```python
from build123d import *

# Parameters (mm, degrees)
BOSS_EXTRUDE1_DEPTH = 185
MIRROR3_START       = -185
MIRROR3_DEPTH       = 370


# Read off the part's stored shape, not the designer's step: Mirror3
with BuildPart() as part:
    # Sketch3 → Boss-Extrude1 (new, symmetric)
    with BuildSketch(Plane.XY):
        with BuildLine():
            Line((0, 8), (0, 3.5))
            ThreePointArc((0, 3.5), (-2.474873734, 2.474873734), (-3.5, 0))
            Line((-3.5, 0), (-8, 0))
            Line((-8, 0), (-8, 4.600266817))
            ThreePointArc((-8, 4.600266817), (-8.096672994, 5.086274776), (-8.371974388, 5.498292429))
            Line((-8.371974388, 5.498292429), (-13.873681959, 11))
            Line((-13.873681959, 11), (-17.7902, 11))
            Line((-17.7902, 11), (-17.7902, 6.2098))
            Line((-17.7902, 6.2098), (-17.0282, 6.2098))
            Line((-17.0282, 6.2098), (-17.0282, 4.508))
            ThreePointArc((-17.0282, 4.508), (-17.176989755, 4.148789755), (-17.5362, 4))
            Line((-17.5362, 4), (-18.8951, 4))
            ThreePointArc((-18.8951, 4), (-19.676382283, 4.323617717), (-20, 5.1049))
            Line((-20, 5.1049), (-20, 16.68))
            ThreePointArc((-20, 16.68), (-19.027594514, 19.027594514), (-16.68, 20))
            Line((-16.68, 20), (-5.1049, 20))
            ThreePointArc((-5.1049, 20), (-4.323617717, 19.676382283), (-4, 18.8951))
            Line((-4, 18.8951), (-4, 17.5362))
            ThreePointArc((-4, 17.5362), (-4.148789755, 17.176989755), (-4.508, 17.0282))
            Line((-4.508, 17.0282), (-6.2098, 17.0282))
            Line((-6.2098, 17.0282), (-6.2098, 17.7902))
            Line((-6.2098, 17.7902), (-11, 17.7902))
            Line((-11, 17.7902), (-11, 13.873681959))
            Line((-11, 13.873681959), (-5.498292429, 8.371974388))
            ThreePointArc((-5.498292429, 8.371974388), (-5.086274776, 8.096672994), (-4.600266817, 8))
            Line((-4.600266817, 8), (0, 8))
        make_face()
        with BuildLine():
            Line((-12.065, 18.73), (-12.065, 12.065))
            Line((-12.065, 12.065), (-18.73, 12.065))
            Line((-18.73, 12.065), (-18.73, 16.19))
            ThreePointArc((-18.73, 16.19), (-17.986051224, 17.986051224), (-16.19, 18.73))
            Line((-16.19, 18.73), (-12.065, 18.73))
        make_face(mode=Mode.SUBTRACT)
    extrude(amount=BOSS_EXTRUDE1_DEPTH, both=True)

    # Mirror1: part across plane


with BuildPart() as part_1:
    add(part.part)
    add(part.part.mirror(Plane(origin=(0, 0, 185), x_dir=(0, 0, 1), z_dir=(1, 0, 0))))

    # Mirror3 outline → Mirror3 (add)
    with BuildSketch(Plane.XY.offset(MIRROR3_START)):
        with BuildLine():
            Line((-8, 0), (-8, -4.600266817))
            ThreePointArc((-8, -4.600266817), (-8.096672994, -5.086274776), (-8.371974388, -5.498292429))
            Line((-8.371974388, -5.498292429), (-13.873681959, -11))
            Line((-13.873681959, -11), (-17.7902, -11))
            Line((-17.7902, -11), (-17.7902, -6.2098))
            Line((-17.7902, -6.2098), (-17.0282, -6.2098))
            Line((-17.0282, -6.2098), (-17.0282, -4.508))
            ThreePointArc((-17.0282, -4.508), (-17.176989755, -4.148789755), (-17.5362, -4))
            Line((-17.5362, -4), (-18.8951, -4))
            ThreePointArc((-18.8951, -4), (-19.676382283, -4.323617717), (-20, -5.1049))
            Line((-20, -5.1049), (-20, -16.68))
            ThreePointArc((-20, -16.68), (-19.027594514, -19.027594514), (-16.68, -20))
            Line((-16.68, -20), (-5.1049, -20))
            ThreePointArc((-5.1049, -20), (-4.323617717, -19.676382283), (-4, -18.8951))
            Line((-4, -18.8951), (-4, -17.5362))
            ThreePointArc((-4, -17.5362), (-4.148789755, -17.176989755), (-4.508, -17.0282))
            Line((-4.508, -17.0282), (-6.2098, -17.0282))
            Line((-6.2098, -17.0282), (-6.2098, -17.7902))
            Line((-6.2098, -17.7902), (-11, -17.7902))
            Line((-11, -17.7902), (-11, -13.873681959))
            Line((-11, -13.873681959), (-5.498292429, -8.371974388))
            ThreePointArc((-5.498292429, -8.371974388), (-5.086274776, -8.096672994), (-4.600266817, -8))
            Line((-4.600266817, -8), (4.600266817, -8))
            ThreePointArc((4.600266817, -8), (5.086274776, -8.096672994), (5.498292429, -8.371974388))
            Line((5.498292429, -8.371974388), (11, -13.873681959))
            Line((11, -13.873681959), (11, -17.7902))
            Line((11, -17.7902), (6.2098, -17.7902))
            Line((6.2098, -17.7902), (6.2098, -17.0282))
            Line((6.2098, -17.0282), (4.508, -17.0282))
            ThreePointArc((4.508, -17.0282), (4.148789755, -17.176989755), (4, -17.5362))
            Line((4, -17.5362), (4, -18.8951))
            ThreePointArc((4, -18.8951), (4.323617717, -19.676382283), (5.1049, -20))
            Line((5.1049, -20), (16.68, -20))
            ThreePointArc((16.68, -20), (19.027594514, -19.027594514), (20, -16.68))
            Line((20, -16.68), (20, -5.1049))
            ThreePointArc((20, -5.1049), (19.676382283, -4.323617717), (18.8951, -4))
            Line((18.8951, -4), (17.5362, -4))
            ThreePointArc((17.5362, -4), (17.176989755, -4.148789755), (17.0282, -4.508))
            Line((17.0282, -4.508), (17.0282, -6.2098))
            Line((17.0282, -6.2098), (17.7902, -6.2098))
            Line((17.7902, -6.2098), (17.7902, -11))
            Line((17.7902, -11), (13.873681959, -11))
            Line((13.873681959, -11), (8.371974388, -5.498292429))
            ThreePointArc((8.371974388, -5.498292429), (8.096672994, -5.086274776), (8, -4.600266817))
            Line((8, -4.600266817), (8, 0))
            Line((8, 0), (3.5, 0))
            ThreePointArc((3.5, 0), (0, -3.5), (-3.5, 0))
            Line((-3.5, 0), (-8, 0))
        make_face()
        with BuildLine():
            Line((-12.065, -12.065), (-12.065, -18.73))
            Line((-12.065, -18.73), (-16.19, -18.73))
            ThreePointArc((-16.19, -18.73), (-17.986051224, -17.986051224), (-18.73, -16.19))
            Line((-18.73, -16.19), (-18.73, -12.065))
            Line((-18.73, -12.065), (-12.065, -12.065))
        make_face(mode=Mode.SUBTRACT)
        with BuildLine():
            Line((12.065, -18.73), (12.065, -12.065))
            Line((12.065, -12.065), (18.73, -12.065))
            Line((18.73, -12.065), (18.73, -16.19))
            ThreePointArc((18.73, -16.19), (17.986051224, -17.986051224), (16.19, -18.73))
            Line((16.19, -18.73), (12.065, -18.73))
        make_face(mode=Mode.SUBTRACT)
    extrude(amount=MIRROR3_DEPTH)


solid = part_1.part
```
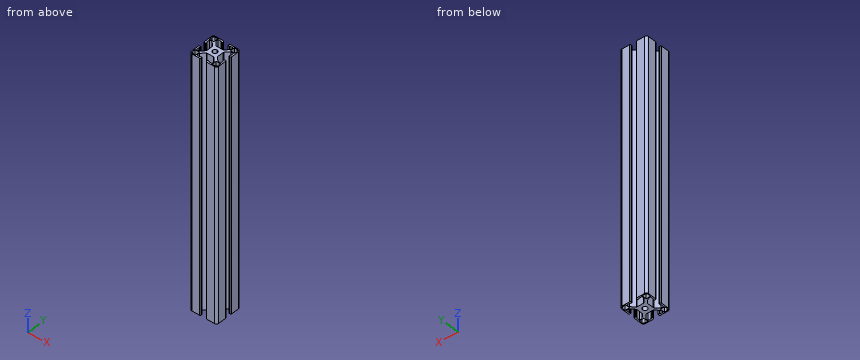
Can you work these out from the model? Positions are in its coordinate system, mm. Give positions to 0.01 mm unless a question says otherwise; leave off trailing zeros. Use a Markdown table: item, result. Add a question column.
Q1. Please list where these lines run through material, in increasing order: line 1 along Y through (x, z) = (-5, 58) (3 decimals); line 2 along Y through (x, z) = (0.5, -85.5); line 3 along Y through (x, z) = (-6, 64.5).
Q2. If we section it at A-A on z = 25: Count the separate pieces of the cut face and the enclosed holes in it, plus the area to 3 significant figures.
Q3. I'm going to push flat-ended pins straight in: pin 1 (1.5 mm diameter, centred on x = 18.5, z = -29, fed in from +Y); pin 2 (2 mm diameter, centred on x = -2.5, z = -113.5, fed in from -Y); pin 3 (0.6 mm diameter, centred on y = -17.5, z = 21.5, fed in from -X). Where does each tip first touch, or does it pass through?
Answers follow:
| question | item | result |
|---|---|---|
| 1 | line 1 | y = -19.995 to -17.028, -8.065 to 8.065, 17.028 to 19.995 |
| 1 | line 2 | y = -8 to -3.46, 3.46 to 8 |
| 1 | line 3 | y = -20 to -17.03, -8.87 to 8.87, 17.03 to 20 |
| 2 | separate pieces | 1 |
| 2 | enclosed holes | 5 |
| 2 | area | 597 mm^2 |
| 3 | pin 1 | stops at y = 19.82 |
| 3 | pin 2 | stops at y = -8 |
| 3 | pin 3 | stops at x = -19.96 |
